Work out the finished part from the listing and answer in its coordinate system (mm). A direction names the side the tool comes from. Coordinates: 2 decimals unless noted, no trailing zeros. Loops run counter-clockwise (first coordinate to the right, second up) from the corner with the lowest first, then second, coordinate; pieces in that order, holes last. Notation, with made-up numbers: (75.5, 39) - (107.5, 39) arc R3 ccw to (107.5, 43) - close; hole circle Ø3 at (44, 74.25). An arc over 180 degrees is marked (long way). Write each question's results on one line, items separated by ' | '. Start each with the question number.
1. A cutting plane is placed at A-A on x = 15.5. Determine the outline of the cut face in (y, z), then the cut area to 3 significant figures.
2. Each of these flat-tipped pins is pushed along its axis until it touches: P1, Ø3.5, axis at x = 15.5, z = 44.5, coming from the +Y side; P2, Ø4.5, axis at x = 15.5, z = 75.5, coming from the +Y side. Where does it stop, or does it pass through?
3. Which of the six approach directions +Z, -Z, +X, -X, +Y, -Y give full straight-line access (tool end or side, diameter ignored) to faces 5 (the cylindrical face through (15.76, -11.96, 73.517)), 6 (the flat face through (23.9, 0, 44))?
4. Determine the mould class of faces 1 (the cylindrical face through (2.493, 11.939, 71.227)), 2 (the flat face through (0, -12, 0)), 3 (the cylindrical face through (-15.066, -11.96, 46.452)), 4 (the flat face through (-25.4, 0, 44)) for opening direction Z: released by +Z, released by -Z, zero draft, split by the parting line, or undercut.
5. A cutting plane is placed at C-C on y = 9. Determine the outline of the cut face in (x, z).
6. A cutting plane is placed at B-B on z = 75.5. Determine the outline of the cut face in (x, y).
7. Find the intervals of material crossed by line 1 along X through (y, z) = (-12.1, 75.5); line 2 along Z through (x, y) = (15.5, -12.25); line 3 along Y through (x, z) = (17, 6), in increasing order. Write a range as [from, to].
8. A cutting plane is placed at D-D on x = -12.5. Determine the outline of the cut face in (y, z), then the cut area to 3 significant figures.
from build123d import *

# Parameters (mm, degrees)
CROQUIS1_W              = 50.8
CROQUIS1_H              = 25.4
CROQUIS1_W_2            = 47.8
CROQUIS1_H_2            = 22.4
SALIENTE_EXTRUIR1_DEPTH = 90
CROQUIS2_R              = 11.5
CROQUIS2_R_2            = 2
CORTAR_EXTRUIR1_DEPTH   = 26


with BuildPart() as part:
    # Croquis1 → Saliente-Extruir1 (new body)
    with BuildSketch(Plane.XY):
        Rectangle(CROQUIS1_W, CROQUIS1_H)
        Rectangle(CROQUIS1_W_2, CROQUIS1_H_2, mode=Mode.SUBTRACT)
    extrude(amount=SALIENTE_EXTRUIR1_DEPTH)

    # Croquis2 → Cortar-Extruir1 (cut)
    with BuildSketch(Plane(origin=(0, -12.7, 0), x_dir=(-1, 0, 0), z_dir=(0, -1, 0))):
        with Locations((0, -60)):
            Circle(CROQUIS2_R)
        with Locations((15.5, -75.5)):
            Circle(CROQUIS2_R_2)
        with Locations((-15.5, -75.5)):
            Circle(CROQUIS2_R_2)
        with Locations((-15.5, -44.5)):
            Circle(CROQUIS2_R_2)
        with Locations((15.5, -44.5)):
            Circle(CROQUIS2_R_2)
    extrude(amount=-CORTAR_EXTRUIR1_DEPTH, mode=Mode.SUBTRACT)


solid = part.part
Values:
1) outline: (-12.7, 0) - (-11.2, 0) - (-11.2, 42.5) - (-12.7, 42.5) - close; (-12.7, 46.5) - (-11.2, 46.5) - (-11.2, 73.5) - (-12.7, 73.5) - close; (-12.7, 77.5) - (-11.2, 77.5) - (-11.2, 90) - (-12.7, 90) - close; (11.2, 0) - (12.7, 0) - (12.7, 42.5) - (11.2, 42.5) - close; (11.2, 46.5) - (12.7, 46.5) - (12.7, 73.5) - (11.2, 73.5) - close; (11.2, 77.5) - (12.7, 77.5) - (12.7, 90) - (11.2, 90) - close | area: 246 mm^2
2) P1: through | P2: y = 12.7
3) face 5: +Y, -Y | face 6: +Z, -Z
4) face 1: undercut | face 2: released by -Z | face 3: undercut | face 4: zero draft
5) outline: (-25.4, 0) - (-23.9, 0) - (-23.9, 90) - (-25.4, 90) - close; (23.9, 0) - (25.4, 0) - (25.4, 90) - (23.9, 90) - close
6) outline: (-25.4, -12.7) - (-17.5, -12.7) - (-17.5, -11.2) - (-23.9, -11.2) - (-23.9, 11.2) - (-17.5, 11.2) - (-17.5, 12.7) - (-25.4, 12.7) - close; (-13.5, -12.7) - (13.5, -12.7) - (13.5, -11.2) - (-13.5, -11.2) - close; (-13.5, 11.2) - (13.5, 11.2) - (13.5, 12.7) - (-13.5, 12.7) - close; (17.5, -12.7) - (25.4, -12.7) - (25.4, 12.7) - (17.5, 12.7) - (17.5, 11.2) - (23.9, 11.2) - (23.9, -11.2) - (17.5, -11.2) - close
7) line 1: [-25.4, -17.5], [-13.5, 13.5], [17.5, 25.4] | line 2: [0, 42.5], [46.5, 73.5], [77.5, 90] | line 3: [-12.7, -11.2], [11.2, 12.7]
8) outline: (-12.7, 0) - (-11.2, 0) - (-11.2, 90) - (-12.7, 90) - close; (11.2, 0) - (12.7, 0) - (12.7, 90) - (11.2, 90) - close | area: 270 mm^2
